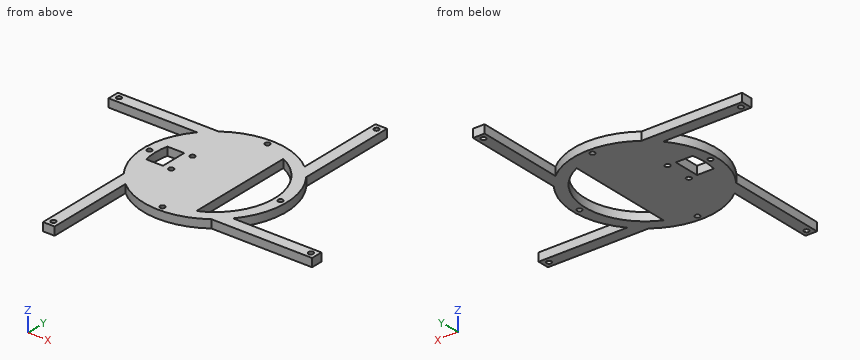
Autodesk Fusion 360 part; units mm, degrees
sketch "スケッチ1" plane through (0, 0, 0) normal (0, 0, 1) x (1, 0, 0)
  circle A0 centre (0, 0) radius 37
  circle A1 centre (0, 0) radius 42
  line L0 (0, 65) -> (28.613, 65)
  line L1 (50, 0) -> (50, -28.613)
  line L2 (0, -50) -> (-28.613, -50)
  line L3 (-50, 0) -> (-50, 28.613)
  line L4 (-50, 28.613) -> (-30.7457, 28.613)
  line L5 (-30.7457, 28.613) -> (-85.2927, 28.613)
  line L6 (-28.613, -50) -> (-28.613, -30.7457)
  line L7 (-28.613, -30.7457) -> (-28.613, -85.2927)
  line L8 (50, -28.613) -> (30.7457, -28.613)
  line L9 (30.7457, -28.613) -> (85.2927, -28.613)
  line L10 (28.613, 65) -> (28.613, 30.7457)
  line L11 (28.613, 30.7457) -> (28.613, 85.2927)
  line L12 (-85.2927, 28.613) -> (-85.2927, 33.613)
  line L13 (-85.2927, 33.613) -> (-25.1827, 33.613)
  line L14 (28.613, 85.2927) -> (33.613, 85.2927)
  line L15 (33.613, 85.2927) -> (33.613, 25.1827)
  line L16 (85.2927, -28.613) -> (85.2927, -33.613)
  line L17 (85.2927, -33.613) -> (25.1827, -33.613)
  line L18 (-28.613, -85.2927) -> (-33.613, -85.2927)
  line L19 (-33.613, -85.2927) -> (-33.613, -25.1827)
  line L20 (-85.2927, 33.613) -> (-80.2927, 33.613)
  line L21 (-85.2927, 31.113) -> (-82.7927, 31.113)
  circle A2 centre (-82.7927, 31.113) radius 1.5
  line L22 (31.113, 85.2927) -> (31.113, 82.7927)
  circle A3 centre (31.113, 82.7927) radius 1.5
  line L23 (85.2927, -31.113) -> (82.7927, -31.113)
  line L24 (-31.113, -85.2927) -> (-31.113, -82.7927)
  circle A4 centre (-31.113, -82.7927) radius 1.5
  circle A5 centre (82.7927, -31.113) radius 1.5
  dimension "d1" = 74
  dimension "d2" = 84
  dimension "d3" = 28.613
  dimension "d4" = 28.613
  dimension "d5" = 28.613
  dimension "d6" = 28.613
  dimension "d7" = 54.547
  dimension "d8" = 54.547
  dimension "d9" = 54.547
  dimension "d10" = 54.547
  dimension "d11" = 5
  dimension "d12" = 5
  dimension "d13" = 5
  dimension "d14" = 5
  dimension "d15" = 5
  dimension "d16" = 3
  dimension "d17" = 2.5
  dimension "d18" = 3
  dimension "d19" = 2.5
  dimension "d20" = 2.5
  dimension "d21" = 3
  dimension "d22" = 3
extrude "押し出し1" add sketch "スケッチ1" along normal blind 3
sketch "スケッチ2" plane through (0, 0, 0) normal (0, 0, 1) x (1, 0, 0)
  line L0 (0, 0) -> (0, 37)
  line L1 (0, 0) -> (37, 0)
  line L2 (0, 0) -> (-37, 0)
  line L3 (0, 0) -> (0, -37)
  line L4 (-37, 0) -> (-39.5, 0)
  line L5 (0, 37) -> (0, 39.5)
  line L6 (37, 0) -> (39.5, 0)
  line L7 (0, -37) -> (0, -39.5)
  circle A0 centre (0, -39.5) radius 1.5
  circle A1 centre (-39.5, 0) radius 1.5
  circle A2 centre (0, 39.5) radius 1.5
  circle A3 centre (39.5, 0) radius 1.5
  dimension "d25" = 37
  dimension "d26" = 37
  dimension "d27" = 37
  dimension "d28" = 37
  dimension "d30" = 2.5
  dimension "d31" = 2.5
  dimension "d32" = 2.5
  dimension "d33" = 2.5
  dimension "d34" = 3
  dimension "d35" = 3
  dimension "d36" = 3
  dimension "d37" = 3
extrude "押し出し2" cut sketch "スケッチ2" along normal blind 3
sketch "スケッチ3" plane through (0, 0, 0) normal (0, 0, 1) x (1, 0, 0)
  line L0 (-31.1, -82.8) -> (-31.1, -83.7)
  line L1 (-31.1, -82.8) -> (-31.1, -86.8)
  line L2 (-31.1, -86.8) -> (-27.1, -86.8)
sketch "スケッチ4" plane through (0, 0, 0) normal (0, 0, 1) x (1, 0, 0)
  circle A0 centre (-82.8, 31.1) radius 1.5
  line L0 (-82.8, 27.6) -> (-86.3, 27.6)
  line L1 (-86.3, 27.6) -> (-86.3, 34.6)
  line L2 (-86.3, 34.6) -> (-82.8171, 34.6)
  line L3 (-39.5, 0) -> (-36, 0)
  line L4 (-39.5, 0) -> (-43, 0)
  circle A1 centre (0, 0) radius 36
  line L5 (31.1, 82.8) -> (34.6, 82.8)
  line L6 (34.6, 82.8) -> (34.6, 86.3)
  line L7 (34.6, 86.3) -> (27.6, 86.3)
  line L8 (82.8, -31.1) -> (86.3, -31.1)
  line L9 (86.3, -31.1) -> (86.3, -34.6)
  line L10 (86.3, -31.1) -> (86.3, -27.6)
  line L11 (-31.1, -82.8) -> (-31.1, -86.8)
  line L12 (-31.1, -82.8) -> (-31.1, -86.3)
  line L13 (-31.1, -86.3) -> (-27.6, -86.3)
  line L14 (-31.1, -86.3) -> (-34.6, -86.3)
  line L15 (-82.8, 27.6) -> (-32.9733, 27.6)
  line L16 (-82.8171, 34.6) -> (-25.5312, 34.6)
  line L17 (27.6, 86.3) -> (27.6, 85.5502)
  line L18 (27.6, 85.5502) -> (27.6, 32.9733)
  line L19 (34.6, 82.8) -> (34.6, 25.5312)
  line L20 (86.3, -27.6) -> (32.9733, -27.6)
  line L21 (86.3, -34.6) -> (25.5312, -34.6)
  line L22 (-27.6, -86.3) -> (-27.6, -32.9733)
  line L23 (-34.6, -86.3) -> (-34.6, -25.5312)
  arc A2 (-32.9733, 27.6) -> (-34.6, -25.5312) centre (0, 0) ccw
  arc A3 (27.6, 32.9733) -> (-25.5312, 34.6) centre (0, 0) ccw
  arc A4 (32.9733, -27.6) -> (34.6, 25.5312) centre (0, 0) ccw
  arc A5 (-27.6, -32.9733) -> (25.5312, -34.6) centre (0, 0) ccw
  circle A6 centre (0, 0) radius 42
  circle A7 centre (0, 0) radius 37
  line L24 (-82.8, 31.1) -> (-82.8, 28.6)
  line L25 (-82.8, 28.6) -> (-30.7578, 28.6)
  line L26 (-82.8, 31.1) -> (-82.8, 33.6)
  circle A8 centre (-31.1, -82.8) radius 1.5
  circle A9 centre (82.8, -31.1) radius 1.5
  circle A10 centre (31.1, 82.8) radius 1.5
  circle A11 centre (39.5, 0) radius 1.5
  circle A12 centre (0, 39.5) radius 1.5
  circle A13 centre (-39.5, 0) radius 1.5
  circle A14 centre (0, -39.5) radius 1.5
  dimension "d40" = 7
  dimension "d42" = 7
  dimension "d43" = 84
  dimension "d44" = 2.5
  dimension "d45" = 3
extrude "押し出し3" add sketch "スケッチ4" against normal blind 5 contours L0 L1 L2 L6 L7 L9 L10 L13 L14 L15 L16 L17 L18 L19 L20 L21 L22 L23 A2 A3 A4 A5 | A7 | A6
extrude "押し出し4" cut 1 faces at (-45.9464, 31.5175, 3) along direction (0, 0, -1) blind 3
sketch "スケッチ5" plane through (0, 0, 0) normal (0, 0, 1) x (1, 0, 0)
  line L0 (15, 33) -> (15, -33)
  arc A0 (15, 32.7261) -> (15, -32.7261) centre (0, 0) ccw
  dimension "d50" = 36
extrude "押し出し5" add sketch "スケッチ5" against normal blind 5
sketch "スケッチ6" plane through (0, 0, 0) normal (0, 0, 1) x (1, 0, 0)
  line L0 (0, 0) -> (-20, 0)
  circle A0 centre (-20, -8) radius 1.5
  circle A1 centre (-20, 8) radius 1.5
  circle A2 centre (0, 0) radius 36
  line L1 (-20, -8) -> (-35.0999, -8)
  line L2 (-20, 8) -> (-35.0999, 8)
  line L3 (-20, -8) -> (-25, -8)
  line L4 (-25, 8) -> (-25, -8)
  dimension "d53" = 8
  dimension "d54" = 8
  dimension "d55" = 3
  dimension "d56" = 3
extrude "押し出し6" cut sketch "スケッチ6" against normal blind 5 contours A0 | A1 | A2 L1 L2 L4 picked at (-28.6332, 0.8955)
Design review of the part built by this model. Coordinates are the model's own, in mm. Give positions to 0.01 mm unless a question says otherwise; leave off trailing zeros. Order: outer loops, then holes, each group sorted by start corner. A loop starts at its lowest first (then second) coordinate and runs counter-clockwise, first axis right, second up. Notation, with made-up numbers: (-6, 66.5) - (41, 66.5) arc R32 cw to (41, 99.5) - close; hole circle Ø9 at (16, -31.5). An arc over 180 degrees is marked (long way). Use CSV: the item, a comma, the result in double quotes. Start each with the question number.
Q1. For P1, Ø2.5, axis at y = 49.5, z = -2.5, coming from the +X side; P2, Ø1.5, axis at y = 7.5, z = -3, coming from the +X side; P3, Ø1.5, axis at x = -44.5, z = -1.5, coming from the +Y side; P4, Ø12, axis at x = 49.5, y = -4.5, coming from the -Z side, all flat-tipped, find the tip position at first contact; note any pin that passes through.
Q2. For line 1 (Y direction, x = 0, z = -3.75); line 2 (X direction, y = 82.8, z = -3.1); line 3 (Y direction, x = 38.5, z = -0.75), list the stretches that pass through material, from the lowest coordinate up.
Q3. Take a section at A-A (y = -20). State the section outline as (x, z) points, and give its area (3 significant figures).
Q4. Take a section at C-C (x = 5). State the section outline as (y, z) points.
Q5. Take a section at B-B (z = -2.85). Count the separate pieces of the cut face and the enclosed holes in it, and give its area (3 significant figures).
Calculated:
1,P1,"stops at x = 34.6"
1,P2,"stops at x = 42.47"
1,P3,"stops at y = 34.6"
1,P4,"passes through"
2,line 1,"y = -43 to -41, -38 to 38, 41 to 43"
2,line 2,"x = 27.6 to 29.6, 32.6 to 34.6"
2,line 3,"y = -34.6 to -27.6, -19.15 to -1.12, 1.12 to 19.15"
3,outline,"(-38.07, -5) - (15, -5) - (15, 0) - (-38.07, 0) - close; (29.93, -5) - (38.07, -5) - (38.07, 0) - (29.93, 0) - close"
3,area,"306 mm²"
4,outline,"(-42.71, -5) - (42.71, -5) - (42.71, 0) - (-42.71, 0) - close"
5,separate pieces,"1"
5,enclosed holes,"12"
5,area,"6,170 mm²"
